Check sheet for the drawn part. Datum: minimum x, y, z corner. Units: mm. A direction names the side the tool comes from. Coordinates: 2 decimals unless noted, no trailing zeros. Order: outer loops, then holes, each group sorted by start corner. A loop starts at its lowest first (then second) coordinate and runs counter-clockwise, first axis right, second up. Notation, with made-up numbers: (85, 34.5) - (121, 34.5) arc R25 ccw to (121, 65.5) - close; hole circle Ø5 at (-2, 76). An arc over 180 degrees is marked (long way). Put each result on its own line as item: value.
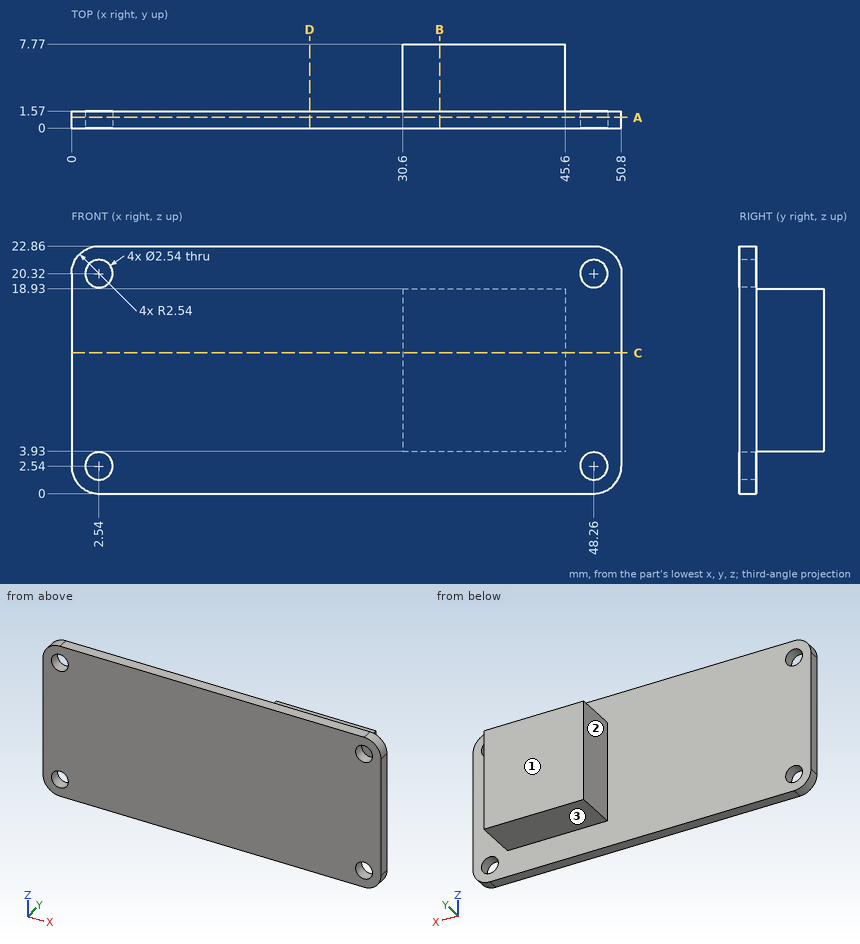
Q1. Section check D-D on x = 22. Record the boundary of the cut face in (y, z), then the cut area to 3 significant figures.
Answer block:
outline: (0, 0) - (1.57, 0) - (1.57, 22.86) - (0, 22.86) - close
area: 35.9 mm^2
Q2. Section check B-B on x = 34. Record the boundary of the cut face in (y, z), then the cut area to 3 significant figures.
Answer block:
outline: (0, 0) - (1.57, 0) - (1.57, 3.93) - (7.77, 3.93) - (7.77, 18.93) - (1.57, 18.93) - (1.57, 22.86) - (0, 22.86) - close
area: 129 mm^2
Q3. Depth check by flat-ended pin: pin 1 Ø3 at (x, y) = (38, 6) entering from +Z; pin 2 Ø2 at (y, z) = (3, 18) entering from -X; pin 3 Ø1 at (x, z) = (37, 14.5) entering from -Y; pin 4 Ø1.9 at (y, z) = (6, 10) entering from +X. Enter the tip coordinate at first touch or a pass-through.
Answer block:
pin 1: stops at z = 18.93
pin 2: stops at x = 30.6
pin 3: stops at y = 0
pin 4: stops at x = 45.6
Q4. Thickness scan on L1, parallel to X at y = 1.2, z = 20.32; L2, parallel to X at y = 1, z = 1.5; L3, parallel to Z at x = 3, y = 1. Record the ranges inside material, lowest first. Write a range as [from, to].
Answer block:
L1: x = [0, 1.27], [3.81, 46.99], [49.53, 50.8]
L2: x = [0.22, 1.81], [3.27, 47.53], [48.99, 50.58]
L3: z = [0, 1.36], [3.72, 19.14], [21.5, 22.86]
Q5. Section check C-C on z = 13. Record the boundary of the cut face in (x, y), then the cut area to 3 significant figures.
Answer block:
outline: (0, 0) - (50.8, 0) - (50.8, 1.57) - (45.6, 1.57) - (45.6, 7.77) - (30.6, 7.77) - (30.6, 1.57) - (0, 1.57) - close
area: 173 mm^2
Q6. Access from +Z, -Z, +X, -X, +Y, -Y to the whole of each face (thin tool, end or side, straight path). Record for the marked faces 1, 2 and 3.
Answer block:
face 1: +Z, -Z, +X, -X, +Y
face 2: +Z, -Z, -X, +Y
face 3: -Z, +X, -X, +Y
Q7. Section check A-A on y = 1. Record the boundary of the cut face in (x, z).
Answer block:
outline: (0, 2.54) arc R2.54 ccw to (2.54, 0) - (48.26, 0) arc R2.54 ccw to (50.8, 2.54) - (50.8, 20.32) arc R2.54 ccw to (48.26, 22.86) - (2.54, 22.86) arc R2.54 ccw to (0, 20.32) - close; hole circle Ø2.54 at (2.54, 2.54); hole circle Ø2.54 at (2.54, 20.32); hole circle Ø2.54 at (48.26, 2.54); hole circle Ø2.54 at (48.26, 20.32)
